The figure shows three views and two pictorial views of one solid part (mm, origin at its lowest corner). Answer the questions. A direction names the side the tool comes from. Round coordinates to 2 decimals unless told otherwise and drop trailing zeros. Order: outer loops, then holes, each group sorted by start corner. A loop starts at its lowest first (then second) coordinate and runs counter-clockwise, first axis right, second up. Notation, with made-up numbers: (-34, -33.75) - (23, -33.75) arc R13 ccw to (23, -22.75) - close; hole circle Ø6 at (67, 55). An arc over 180 degrees is marked (long way). Use CSV: the item, a comma, the result in double quotes. Start each with the question number.
Item 1: Find section D-D, the plane x = 13. Give the vertices of the cut face in (y, z).
Item 2: Find section A-A, the plane x = 31. Give the vertices of the cut face in (y, z), plus the area to 3 significant figures.
Item 3: Find section C-C, the plane z = 2.85. Give the vertices of the cut face in (x, y).
Item 4: Straight lines are drawn through the part: line 1 along Y through (x, z) = (5, 1.35); line 2 along Y through (x, z) = (18, 1.4); line 3 along X through (y, z) = (8.5, 2.65). For each, find the intervals that lie inside material, in ascending order. Write a range as [from, to].
Item 5: Flat-ended cylindrical pins translate along their axes: P1, Ø0.5, axis at x = 22.5, z = 3, coming from the -Y side; P2, Ø3, axis at x = 23.5, y = 7, coming from the +Z side. Find the tip coordinate at first contact, or state that the pin passes through.
Item 6: Find section B-B, the plane y = 6.5. Give the vertices of the cut face in (x, z), plus the area to 4 significant figures.
Item 7: For the marked faces 4 and 5, determine the directions among +Z, -Z, +X, -X, +Y, -Y from which every point of the face is accessible in a straight line to the end or side of a thin tool.
Item 8: Determine the mould class of the marked faces 1, 2 and 3 for opening direction Y: +Y half, -Y half, draft (parallel to the pull), parting line (faces both ways), or undercut.
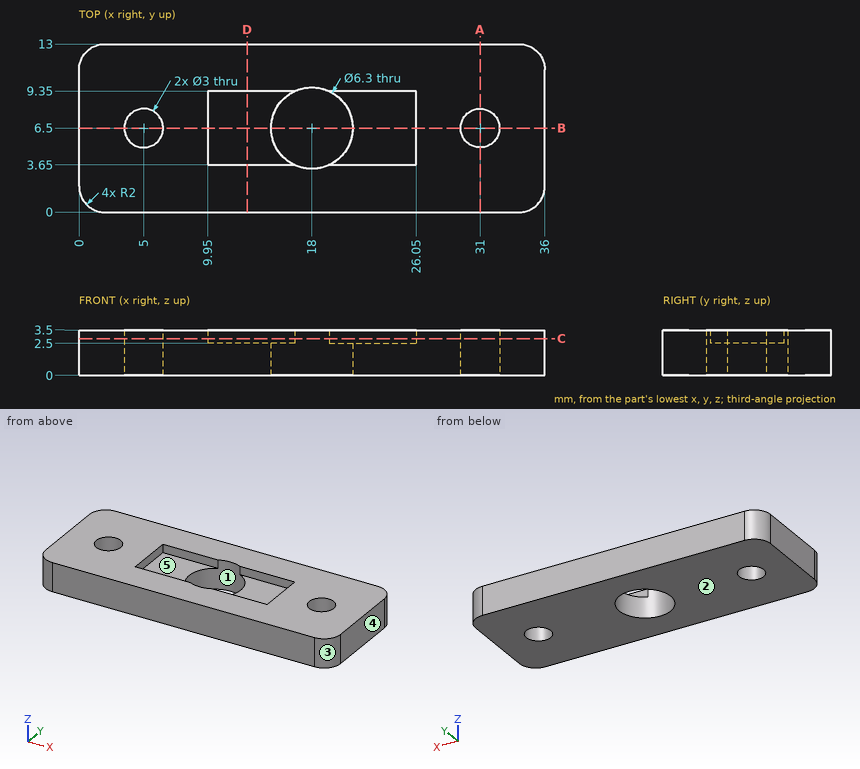
Worked out:
1,outline,"(0, 0) - (13, 0) - (13, 3.5) - (9.35, 3.5) - (9.35, 2.5) - (3.65, 2.5) - (3.65, 3.5) - (0, 3.5) - close"
2,outline,"(0, 0) - (5, 0) - (5, 3.5) - (0, 3.5) - close; (8, 0) - (13, 0) - (13, 3.5) - (8, 3.5) - close"
2,area,"35.0 mm²"
3,outline,"(0, 2) arc R2 ccw to (2, 0) - (34, 0) arc R2 ccw to (36, 2) - (36, 11) arc R2 ccw to (34, 13) - (2, 13) arc R2 ccw to (0, 11) - close; hole circle Ø3 at (5, 6.5); hole (9.95, 3.65) - (16.66, 3.65) arc R3.15 ccw to (19.34, 3.65) - (26.05, 3.65) - (26.05, 9.35) - (19.34, 9.35) arc R3.15 ccw to (16.66, 9.35) - (9.95, 9.35) - close; hole circle Ø3 at (31, 6.5)"
4,line 1,"y = [0, 5], [8, 13]"
4,line 2,"y = [0, 3.35], [9.65, 13]"
4,line 3,"x = [0, 9.95], [26.05, 36]"
5,P1,"stops at y = 0"
5,P2,"stops at z = 2.5"
6,outline,"(0, 0) - (3.5, 0) - (3.5, 3.5) - (0, 3.5) - close; (6.5, 0) - (14.85, 0) - (14.85, 2.5) - (9.95, 2.5) - (9.95, 3.5) - (6.5, 3.5) - close; (21.15, 0) - (29.5, 0) - (29.5, 3.5) - (26.05, 3.5) - (26.05, 2.5) - (21.15, 2.5) - close; (32.5, 0) - (36, 0) - (36, 3.5) - (32.5, 3.5) - close"
6,area,"73.15 mm²"
7,face 4,"+Z, -Z, +X, +Y, -Y"
7,face 5,"+Z"
8,face 1,"undercut"
8,face 2,"draft"
8,face 3,"-Y half"
